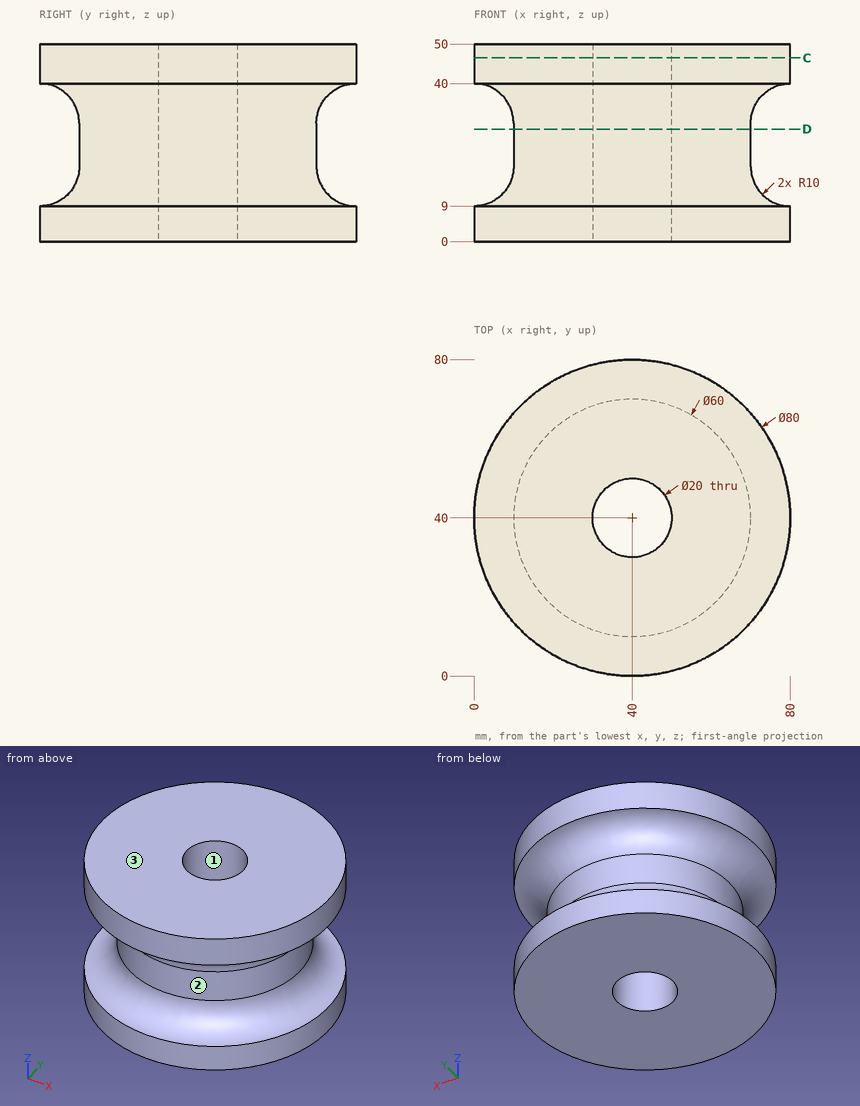
Check sheet for the drawn part. Datum: minimum x, y, z corner. Units: mm. Round coordinates to 2 decimals unless told otherwise and drop trailing zeros. Order: outer loops, then holes, each group sorted by start corner. A loop starts at its lowest first (then second) coordinate and runs counter-clockwise, first axis right, second up. Notation, with made-up numbers: (-15, -1.75) -> (39, -1.75) arc R12 cw to (39, 8.25) -> close; hole circle Ø1 at (12, 11). An arc over 180 degrees is marked (long way). Return JSON: item names as keys, results as strings. Group by question number.
Q1. Section check C-C, the plane z = 46.5. Record the boundary of the cut face in (x, y), plus the area to 3 significant figures.
Q2. Release check for a two-part mould opening along Y. For the marked faces 1, 2 and 3 record: released by +Y, released by -Y, zero draft, split by the parting line, or undercut.
Q3. Section check D-D, the plane z = 28.5. Record the boundary of the cut face in (x, y), plus the area to 3 significant figures.
Q4. Gauge pin test, flat ends, axial feed: pin 1 (1.5 mm diameter, centred on y = 53.5, z = 23, fed in from -X); pin 2 (3 mm diameter, centred on y = 63.5, z = 39.5, fed in from +X); pin 3 (1 mm diameter, centred on x = 13.5, z = 26.5, fed in from -Y). Record the tip position at first contact, or that the pin passes through.
Q5. Material ranges on probe 1 along Y at (x, z) = (40, 21); probe 2 along Y at (x, z) = (40, 13.5); probe 3 along Z at (x, y) = (62.5, 8), recorded low to high. Write a range as from..to.
Numbers:
{
 "1": {"outline": "circle Ø80 at (40, 40); hole circle Ø20 at (40, 40)", "area": "4,710 mm^2"},
 "2": {"face 1": "undercut", "face 2": "split by the parting line", "face 3": "zero draft"},
 "3": {"outline": "circle Ø60 at (40, 40); hole circle Ø20 at (40, 40)", "area": "2,510 mm^2"},
 "4": {"pin 1": "x = 12.84", "pin 2": "x = 73.35", "pin 3": "y = 25.03"},
 "5": {"probe 1": "10..30, 50..70", "probe 2": "8.35..30, 50..71.65", "probe 3": "0..9.04, 39.96..50"}
}
